Geometry check sheet. Reference: drawing and pictorial views, mm from the part's lowest x, y, z. A direction names the side the tool comes from. Round coordinates to 2 decimals unless told otherwise and drop trailing zeros. Order: outer loops, then holes, each group sorted by start corner. A loop starts at its lowest first (then second) coordinate and runs counter-clockwise, first axis right, second up. Notation, with made-up numbers: (82.5, 12) -> (94.5, 12) arc R23 cw to (94.5, 24) -> close; hole circle Ø3 at (-26, 6.25). An arc over 180 degrees is marked (long way). Put each result on its own line as item: value.
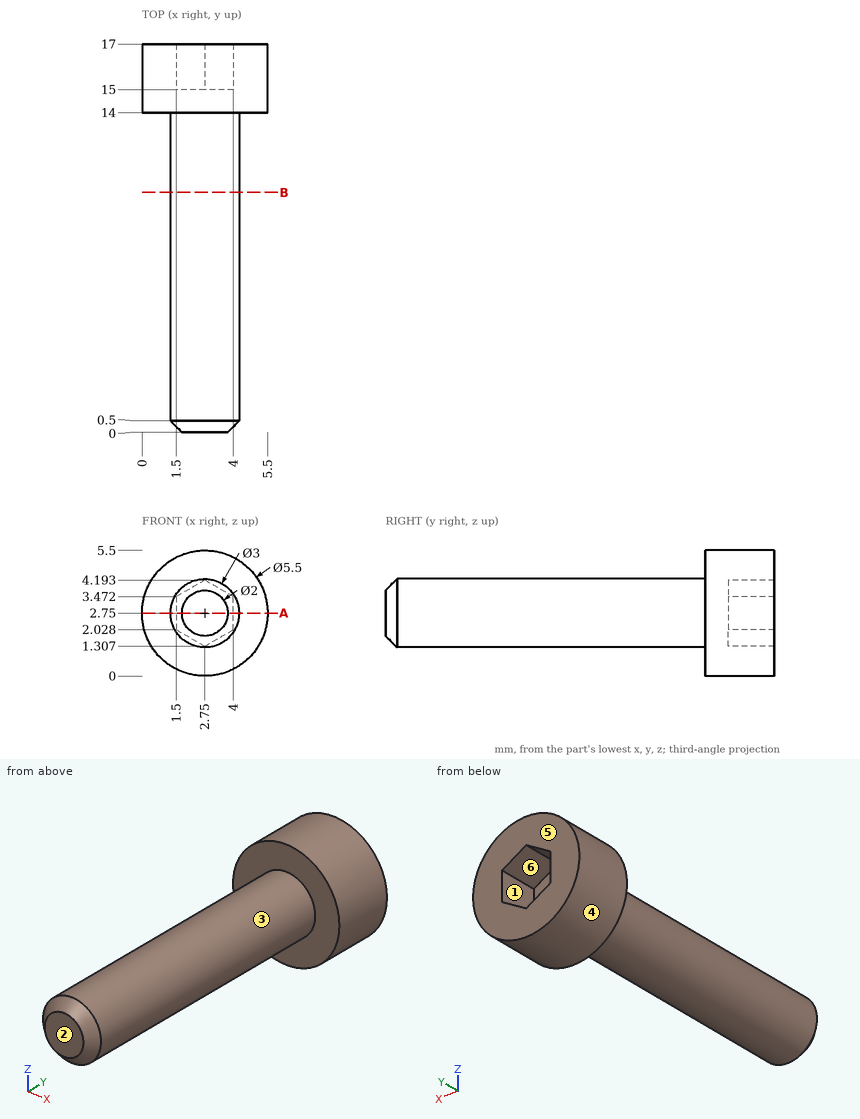
Item 1: Sectioned sample at A-A, the plane z = 2.75. Record the boundary of the cut face in (x, y).
Geometry check:
outline: (0, 14) -> (1.25, 14) -> (1.25, 0.5) -> (1.75, 0) -> (3.75, 0) -> (4.25, 0.5) -> (4.25, 14) -> (5.5, 14) -> (5.5, 17) -> (4, 17) -> (4, 15) -> (1.5, 15) -> (1.5, 17) -> (0, 17) -> close
Item 2: Sectioned sample at B-B, the plane y = 10.5. Record the boundary of the cut face in (x, z).
Geometry check:
outline: circle Ø3 at (2.75, 2.75)
Item 3: Material ranges on line 1 along Y through (x, z) = (3.3, 3.4); line 2 along Y through (x, z) = (2.9, 5.15); line 3 along X through (y, z) = (4.75, 2.8), recorded low to high.
Geometry check:
line 1: 0 to 15
line 2: 14 to 17
line 3: 1.25 to 4.25
Item 4: Depth check by flat-ended pin: pin 1 Ø0.8 at (x, z) = (2.5, 3) entering from +Y; pin 2 Ø1.2 at (y, z) = (16, 3) entering from +X; pin 3 Ø1.5 at (x, y) = (1.5, 10.5) entering from -Z (1 decimal). Enter the tip coordinate at first touch or a pass-through.
Geometry check:
pin 1: y = 15
pin 2: x = 5.5
pin 3: z = 1.3
Item 5: Tool access check on the marked faces 1, 2 and 3. Record the directions out of +Z, -Z, +X, -X, +Y, -Y that give a thin tool (end or side, any length) a straight path to the whole face; none if there is none.
Geometry check:
face 1: +Y
face 2: +Z, -Z, +X, -X, -Y
face 3: -Y
Item 6: Release check for a two-part mould opening along Z. For the marked faces 4, 5 and 6 record: pulls with the +Z half, pulls with the -Z half, needs draft (parallel to the pull), parting line crosses it, or undercut.
Geometry check:
face 4: parting line crosses it
face 5: needs draft
face 6: undercut
